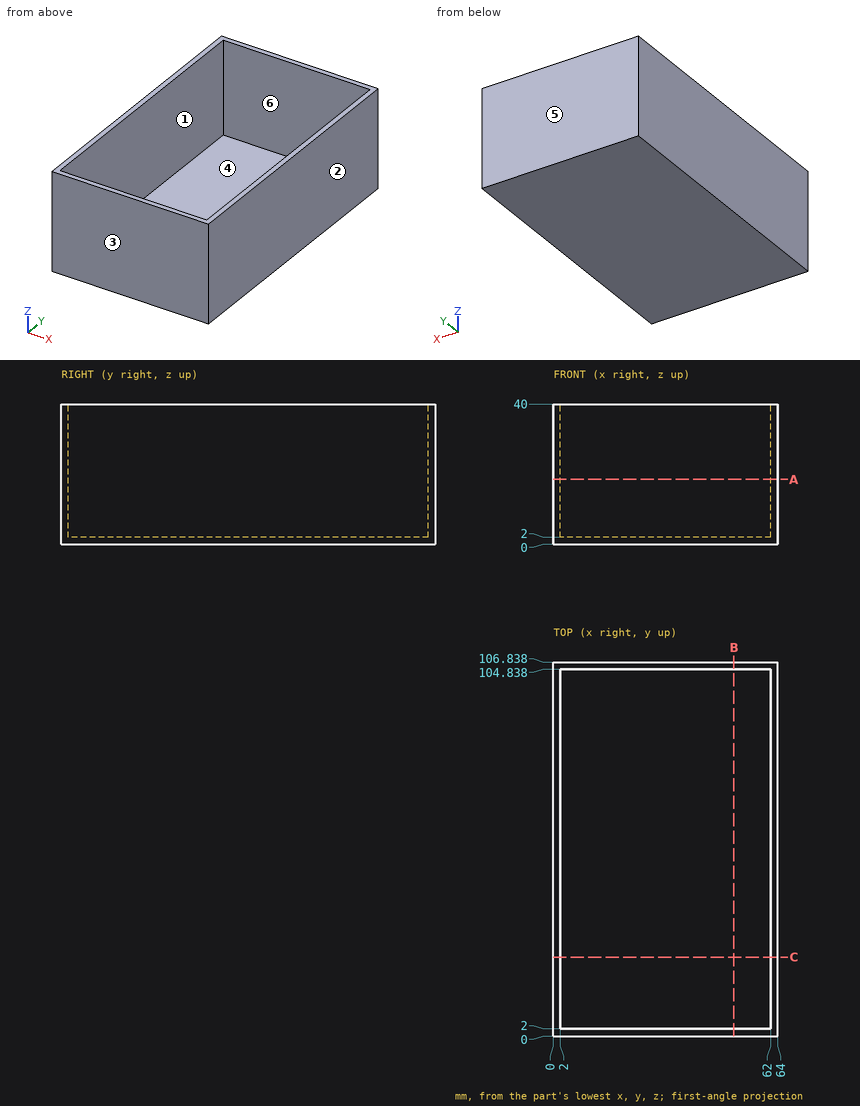
Source: three-view drawing plus pictorial views. Frame: mm from the lowest corner of the part. A direction names the side the tool comes from. Coordinates: 2 decimals unless noted, no trailing zeros. Order: outer loops, then holes, each group sorted by start corner. A loop starts at its lowest first (then second) coordinate and runs counter-clockwise, first axis right, second up.
Item 1: Pull-direction query (X, two-part tool) for the marked faces 1, 2, 3 and 4; classes: pulls with the +X half, pulls with the -X half, needs draft (parallel to the pull), parting line crosses it, or undercut.
Output values:
face 1: undercut
face 2: pulls with the +X half
face 3: needs draft
face 4: undercut
Item 2: First-contact query: P1, Ø6, axis at x = 56.5, y = 12.5, coming from the +Z side. Flat tip, straight axial feed; report the tip coordinate or a pass-through.
Output values:
P1: stops at z = 2
Item 3: Cut plane A-A (z = 18.5). Return loops of the section in (x, y), plus the area to 3 significant figures.
Output values:
outline: (0, 0) - (64, 0) - (64, 106.84) - (0, 106.84) - close; hole (2, 2) - (62, 2) - (62, 104.84) - (2, 104.84) - close
area: 667 mm2
Item 4: Cut plane B-B (x = 51.5). Return loops of the section in (y, z).
Output values:
outline: (0, 0) - (106.84, 0) - (106.84, 40) - (104.84, 40) - (104.84, 2) - (2, 2) - (2, 40) - (0, 40) - close
Item 5: Material intervals for line 1 (Y direction, x = 6.5, z = 25); line 2 (X direction, y = 68.5, z = 2.5); line 3 (Z direction, x = 19, y = 84), sorted ascending.
Output values:
line 1: y = 0 to 2, 104.84 to 106.84
line 2: x = 0 to 2, 62 to 64
line 3: z = 0 to 2
Item 6: Cut plane C-C (y = 22.5). Return loops of the section in (x, z), plus the area to 3 significant figures.
Output values:
outline: (0, 0) - (64, 0) - (64, 40) - (62, 40) - (62, 2) - (2, 2) - (2, 40) - (0, 40) - close
area: 280 mm2
Item 7: Set-up query: the marked faces 5 and 6. Return all of +Z, -Z, +X, -X, +Y, -Y with unobstructed straight access to the full face (end or side cutting, diameter ignored); none if empty.
Output values:
face 5: +Z, -Z, +X, -X, +Y
face 6: +Z
